Autodesk Inventor part; units mm, degrees
ref_plane "YZ Plane" through (0, 0, 0) normal (1, 0, 0) x (0, 1, 0)
ref_plane "XZ Plane" through (0, 0, 0) normal (0, 1, 0) x (-1, 0, 0)
ref_plane "XY Plane" through (0, 0, 0) normal (0, 0, 1) x (1, 0, 0)
sketch "Esboço1" plane through (0, 0, 0) normal (0, 0, 1) x (1, 0, 0)
  line L0 (0, 0) -> (20, 0)
  arc A0 (40, 0) -> (20, 0) centre (30, 0) ccw
  line L1 (40, 0) -> (55, 0)
  line L2 (55, 2) -> (41.8322, 2)
  arc A1 (41.8322, 2) -> (18.1678, 2) centre (30, 0) ccw
  line L3 (18.1678, 2) -> (0, 2)
  line L4 (0, 0) -> (0, 2)
  line L5 (55, 2) -> (55, 0)
  line L6 (-5.5604, -3.5) -> (66.7999, -3.5)
  line L7 (0, -7) -> (20, -7)
  arc A2 (20, -7) -> (40, -7) centre (30, -7) ccw
  line L8 (40, -7) -> (55, -7)
  line L9 (55, -9) -> (41.8322, -9)
  arc A3 (18.1678, -9) -> (41.8322, -9) centre (30, -7) ccw
  line L10 (18.1678, -9) -> (0, -9)
  line L11 (0, -7) -> (0, -9)
  line L12 (55, -9) -> (55, -7)
  line L13 (0, -7) -> (20, -7)
  line L14 (20, -7) -> (20, 0)
  line L15 (20, 0) -> (0, 0)
  line L16 (0, 0) -> (0, -7)
  line L17 (51.1425, 2) -> (44.7734, 2)
  line L18 (44.7734, 2) -> (44.7734, 4)
  line L19 (44.7734, 4) -> (51.1425, 4)
  line L20 (51.1425, 4) -> (51.1425, 2)
  line L21 (51.1425, -9) -> (44.7734, -9)
  line L22 (44.7734, -9) -> (44.7734, -11)
  line L23 (44.7734, -11) -> (51.1425, -11)
  line L24 (51.1425, -11) -> (51.1425, -9)
  point P0 (44.7734, -9)
  point P1 (20, -7)
  dimension "d0" = 20
  dimension "d1" = 20
  dimension "d2" = 10
  dimension "d3" = 15
  dimension "d4" = 2
  dimension "d5" = 7
  dimension "d6" = 2
  dimension "d7" = 2
extrude "Extrusão1" add sketch "Esboço1" along normal blind 15
sketch "Esboço2" plane through (44.7734, 4, 0) normal (0, 1, 0) x (1, 0, 0)
  circle A0 centre (3.195, -7.5) radius 1.5
  line L0 (6.3691, 0) -> (0, 0)
  line L1 (0, 0) -> (0, -15)
  point P0 (-44.7734, 0)
  dimension "d10" = 3
  dimension "d11" = 7.5
  dimension "d12" = 3.195
extrude "Extrusão2" cut sketch "Esboço2" against normal blind 15
sketch "Esboço3" plane through (40, -7, 0) normal (0, 1, 0) x (1, 0, 0)
  circle A0 centre (7.6045, -7.5) radius 5
  circle A1 centre (7.6045, -7.5) radius 6
  point P0 (-40, 0)
  dimension "d15" = 10
  dimension "d16" = 12
extrude "Extrusão3" add sketch "Esboço3" along normal blind 1
sketch "Esboço4" plane through (40, 0, 0) normal (0, -1, 0) x (1, 0, 0)
  circle A0 centre (7.9684, 7.5) radius 1.5
  circle A1 centre (7.9684, 7.5) radius 5
  circle A2 centre (7.9684, 7.5) radius 6
  point P0 (-40, 0)
  dimension "d19" = 10
  dimension "d20" = 12
extrude "Extrusão4" add sketch "Esboço4" along normal blind 1 contours A2
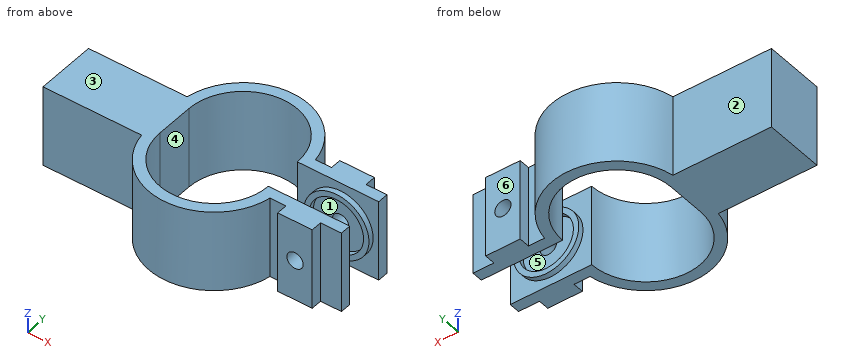
The listing builds one solid part. Answer for the finished solid, in the listing's coordinates (mm). Face numbers are marked on the shaded views. A direction names the side the tool comes from. Coordinates: 2 decimals unless noted, no trailing zeros. Write each loop counter-clockwise with the first axis right and the second up, starting at its lowest first coordinate (ties: lowest second). Pieces come first, ordered by that corner, then holes. Notation, with made-up numbers: (12, -26) - (52, -26) arc R33 ccw to (52, 10) - close; hole circle Ø5 at (74.5, -2). An arc over 180 degrees is marked (long way). One line per item, written item: value.
1) Find section A-A (x = 37). Give the vertices of the cut face in (y, z).
Geometry check:
outline: (-16.75, 0) - (-14.14, 0) - (-14.14, 15) - (-16.75, 15) - close; (7.14, 0) - (9.75, 0) - (9.75, 15) - (7.14, 15) - close
2) Find section B-B (y = 7.5). Give the vertices of the cut face in (x, z), and give its area (3 significant figures).
Geometry check:
outline: (20.63, 0) - (23.39, 0) - (23.39, 15) - (20.63, 15) - close; (36.61, 0) - (39.37, 0) - (39.37, 15) - (36.61, 15) - close
area: 82.6 mm2
3) A tool of negligible diameter and unlimited length cuts with its end or side. For the marked faces 4, 5 and 6, from which of +Z, -Z, +X, -X, +Y, -Y can it reach the whole face along a straight path? Write none if from no direction.
Geometry check:
face 4: +Z, -Z
face 5: none
face 6: +Z, -Z, +X, +Y
4) Find section D-D (x = 11). Give the vertices of the cut face in (y, z), and give its area (3 significant figures).
Geometry check:
outline: (-9, 0) - (2, 0) - (2, 15) - (-9, 15) - close
area: 165 mm2
5) Consider line 1 along X through (y, z) = (-6.6, 7.5); line 2 along Y through (x, z) = (44, 6.75); line 3 along X through (y, z) = (3.2, 7.5). Determine where each line is inside the solid, lowest interval first. Write a range as from..to.
Geometry check:
line 1: x = 0..20, 41.6..42.6, 52.6..53.6
line 2: y = -9..-7, 0..2
line 3: x = 18.43..20.53, 39.47..41.57, 44.77..46.47, 49.47..51.14
6) For a pull along Y with two mould halves and no side action, classify the marked faces 1, 2 and 3 as pulls with the +Y half, pulls with the -Y half, needs draft (parallel to the pull), parting line crosses it, or undercut.
Geometry check:
face 1: undercut
face 2: pulls with the +Y half
face 3: needs draft
7) Find section C-C (z = 7.5). Count the separate pieces of the cut face and the enclosed holes in it, and give its area (3 significant figures).
Geometry check:
separate pieces: 3
enclosed holes: 0
area: 408 mm2
8) Each of these flat-tipped pins is pushed along its axis until it touches: pin 1 Ø1.9 at (x, z) = (53.5, 4) entering from -Y; pin 2 Ø2.5 at (x, z) = (47.97, 7.5) entering from +Y; pin 3 Ø1.6 at (y, z) = (-10, 10) entering from -X; pin 4 Ø4.5 at (x, z) = (51, 5.5) entering from +Y. Where does it stop, or does it pass through?
Geometry check:
pin 1: stops at y = -9
pin 2: passes through
pin 3: stops at x = 18.2
pin 4: stops at y = 4
